Design review of the part built by this model. Coordinates are the model's own, in mm. Coordinates: 2 decimals unless noted, no trailing zeros. Loops run counter-clockwise (first coordinate to the right, second up) from the corner with the lowest first, then second, coordinate; pieces in that order, holes last. Notation, with made-up numbers: (8, 63.25) -> (38, 63.25) arc R21 ccw to (38, 88.25) -> close; hole circle Ø6 at (36.25, 60.5). An arc over 180 degrees is marked (long way). Answer as a JSON object with one key per item and string values.
Autodesk Inventor part; units mm, degrees
ref_plane "Начальная плоскость" through (0, 0, 0) normal (0, 0, 1) x (1, 0, 0)
ref_plane "Конечная плоскость" through (0, 0, 100) normal (0, 0, 1) x (1, 0, 0)
ref_plane "YZ Plane" through (0, 0, 0) normal (1, 0, 0) x (0, 1, 0)
ref_plane "Начальная плоскость" through (0, 0, 0) normal (0, 0, 1) x (1, 0, 0)
ref_plane "Конечная плоскость" through (0, 0, 100) normal (0, 0, 1) x (1, 0, 0)
sketch "Эскиз1" plane through (0, 0, 0) normal (0, 0, 1) x (1, 0, 0)
  line L0 (-14.4349, 0) -> (14.4349, 0)
  line L1 (0, -14) -> (0, 14)
  line L2 (0, 0) -> (7.5, 7.5) construction
  circle A0 centre (7.5, 7.5) radius 1.65 construction
  line L3 (5.85, 9.15) -> (9.15, 9.15)
  line L4 (9.15, 9.15) -> (9.15, 5.85)
  line L5 (9.15, 5.85) -> (5.85, 5.85)
  line L6 (5.85, 5.85) -> (5.85, 9.15)
  line L7 (3.235, 8.1636) -> (4.72, 9.9636)
  line L8 (4.7971, 10) -> (8.5, 10)
  line L9 (3.3121, 8) -> (4.95, 8)
  line L10 (4.95, 8) -> (4.95, 5.7985)
  line L11 (4.95, 5.7985) -> (2.6515, 3.5)
  line L12 (0, 3.5) -> (2.6515, 3.5)
  circle A1 centre (0, 0) radius 2.25
  line L13 (8.1636, 3.235) -> (9.9636, 4.72)
  line L14 (10, 4.7971) -> (10, 8.5)
  line L15 (8, 3.3121) -> (8, 4.95)
  line L16 (8, 4.95) -> (5.7985, 4.95)
  line L17 (5.7985, 4.95) -> (3.5, 2.6515)
  line L18 (3.5, 0) -> (3.5, 2.6515)
  arc A2 (10, 8.5) -> (8.5, 10) centre (8.5, 8.5) ccw
  line L19 (0, 0) -> (-7.5, 7.5) construction
  circle A3 centre (-7.5, 7.5) radius 1.65 construction
  line L20 (-5.85, 9.15) -> (-9.15, 9.15)
  line L21 (-9.15, 9.15) -> (-9.15, 5.85)
  line L22 (-9.15, 5.85) -> (-5.85, 5.85)
  line L23 (-5.85, 5.85) -> (-5.85, 9.15)
  line L24 (-3.235, 8.1636) -> (-4.72, 9.9636)
  line L25 (-4.7971, 10) -> (-8.5, 10)
  line L26 (-3.3121, 8) -> (-4.95, 8)
  line L27 (-4.95, 8) -> (-4.95, 5.7985)
  line L28 (-4.95, 5.7985) -> (-2.6515, 3.5)
  line L29 (0, 3.5) -> (-2.6515, 3.5)
  line L30 (-3.5, 0) -> (-3.5, 2.6515)
  line L31 (-5.7985, 4.95) -> (-3.5, 2.6515)
  line L32 (-8, 4.95) -> (-5.7985, 4.95)
  line L33 (-8, 3.3121) -> (-8, 4.95)
  line L34 (-8.1636, 3.235) -> (-9.9636, 4.72)
  line L35 (-10, 4.7971) -> (-10, 8.5)
  arc A4 (-8.5, 10) -> (-10, 8.5) centre (-8.5, 8.5) ccw
  line L36 (0, 14) -> (0, -14)
  line L37 (0, 0) -> (7.5, -7.5) construction
  circle A5 centre (7.5, -7.5) radius 1.65 construction
  line L38 (5.85, -9.15) -> (9.15, -9.15)
  line L39 (9.15, -9.15) -> (9.15, -5.85)
  line L40 (9.15, -5.85) -> (5.85, -5.85)
  line L41 (5.85, -5.85) -> (5.85, -9.15)
  line L42 (3.235, -8.1636) -> (4.72, -9.9636)
  line L43 (4.7971, -10) -> (8.5, -10)
  line L44 (3.3121, -8) -> (4.95, -8)
  line L45 (4.95, -8) -> (4.95, -5.7985)
  line L46 (4.95, -5.7985) -> (2.6515, -3.5)
  line L47 (0, -3.5) -> (2.6515, -3.5)
  line L48 (3.5, 0) -> (3.5, -2.6515)
  line L49 (5.7985, -4.95) -> (3.5, -2.6515)
  line L50 (8, -4.95) -> (5.7985, -4.95)
  line L51 (8, -3.3121) -> (8, -4.95)
  line L52 (8.1636, -3.235) -> (9.9636, -4.72)
  line L53 (10, -4.7971) -> (10, -8.5)
  arc A6 (8.5, -10) -> (10, -8.5) centre (8.5, -8.5) ccw
  line L54 (0, 0) -> (-7.5, -7.5) construction
  line L55 (-4.95, -8) -> (-4.95, -5.7985)
  line L56 (-3.3121, -8) -> (-4.95, -8)
  line L57 (-5.7985, -4.95) -> (-3.5, -2.6515)
  line L58 (-4.95, -5.7985) -> (-2.6515, -3.5)
  line L59 (-3.5, 0) -> (-3.5, -2.6515)
  line L60 (0, -3.5) -> (-2.6515, -3.5)
  circle A7 centre (-7.5, -7.5) radius 1.65 construction
  line L61 (-5.85, -5.85) -> (-5.85, -9.15)
  line L62 (-5.85, -9.15) -> (-9.15, -9.15)
  line L63 (-9.15, -9.15) -> (-9.15, -5.85)
  line L64 (-9.15, -5.85) -> (-5.85, -5.85)
  line L65 (-3.235, -8.1636) -> (-4.72, -9.9636)
  line L66 (-8, -4.95) -> (-5.7985, -4.95)
  line L67 (-8, -3.3121) -> (-8, -4.95)
  line L68 (-8.1636, -3.235) -> (-9.9636, -4.72)
  line L69 (-4.7971, -10) -> (-8.5, -10)
  line L70 (-10, -4.7971) -> (-10, -8.5)
  arc A8 (-10, -8.5) -> (-8.5, -10) centre (-8.5, -8.5) ccw
  arc A9 (3.235, 8.1636) -> (3.3121, 8) centre (3.3121, 8.1) ccw
  arc A10 (4.7971, 10) -> (4.72, 9.9636) centre (4.7971, 9.9) ccw
  arc A11 (8, 3.3121) -> (8.1636, 3.235) centre (8.1, 3.3121) ccw
  arc A12 (9.9636, 4.72) -> (10, 4.7971) centre (9.9, 4.7971) ccw
  arc A13 (-3.3121, 8) -> (-3.235, 8.1636) centre (-3.3121, 8.1) ccw
  arc A14 (-4.72, 9.9636) -> (-4.7971, 10) centre (-4.7971, 9.9) ccw
  arc A15 (-8.1636, 3.235) -> (-8, 3.3121) centre (-8.1, 3.3121) ccw
  arc A16 (-10, 4.7971) -> (-9.9636, 4.72) centre (-9.9, 4.7971) ccw
  arc A17 (-8, -3.3121) -> (-8.1636, -3.235) centre (-8.1, -3.3121) ccw
  arc A18 (-9.9636, -4.72) -> (-10, -4.7971) centre (-9.9, -4.7971) ccw
  arc A19 (-3.235, -8.1636) -> (-3.3121, -8) centre (-3.3121, -8.1) ccw
  arc A20 (-4.7971, -10) -> (-4.72, -9.9636) centre (-4.7971, -9.9) ccw
  arc A21 (4.72, -9.9636) -> (4.7971, -10) centre (4.7971, -9.9) ccw
  arc A22 (3.3121, -8) -> (3.235, -8.1636) centre (3.3121, -8.1) ccw
  arc A23 (8.1636, -3.235) -> (8, -3.3121) centre (8.1, -3.3121) ccw
  arc A24 (10, -4.7971) -> (9.9636, -4.72) centre (9.9, -4.7971) ccw
  point P0 (3.1, 8)
  point P1 (4.75, 10)
  point P2 (7.5, 9.15)
  point P3 (8, 3.1)
  point P4 (10, 4.75)
  point P5 (7.5, 5.85)
  point P6 (9.15, 7.5)
  point P7 (-3.1, 8)
  point P8 (-4.75, 10)
  point P9 (-7.5, 9.15)
  point P10 (-8, 3.1)
  point P11 (-10, 4.75)
  point P12 (-7.5, 5.85)
  point P13 (-9.15, 7.5)
  point P14 (3.1, -8)
  point P15 (4.75, -10)
  point P16 (7.5, -9.15)
  point P17 (8, -3.1)
  point P18 (10, -4.75)
  point P19 (7.5, -5.85)
  point P20 (9.15, -7.5)
  point P21 (-3.1, -8)
  point P22 (-7.5, -5.85)
  point P23 (-7.5, -9.15)
  point P24 (-9.15, -7.5)
  point P25 (-4.75, -10)
  point P26 (-8, -3.1)
  point P27 (-10, -4.75)
  dimension "d0" = 45
  dimension "d1" = 3.3
  dimension "d2" = 1.5
  dimension "d3" = 1.2
  dimension "d4" = 4.5
  dimension "d5" = 6.5
  dimension "d6" = 15
  dimension "d7" = 20
  dimension "d8" = 9.9
  dimension "d9" = 9.5
  dimension "d10" = 6.2
  dimension "d11" = 2
  dimension "d18" = 0.1
  dimension "d19" = 0.1
extrude "Тело" add sketch "Эскиз1" along normal up to surface (100 mm away) from surface at 0 contours A1 L1 L12 L11 L10 L9 A9 L7 A10 L8 A2 L14 A12 L13 A11 L15 L16 L17 L18 L0 | L0 L48 L49 L50 L51 A23 L52 A24 L53 A6 L43 A21 L42 A22 L44 L45 L46 L47 L1 A1 | A1 L0 L30 L31 L32 L33 A15 L34 A16 L35 A4 L25 A14 L24 A13 L26 L27 L28 L29 L1 | L1 L60 L58 L55 L56 A19 L65 A20 L69 A8 L70 A18 L68 A17 L67 L66 L57 L59 L0 A1
sketch "Эскиз2" plane through (0, 0, 0) normal (0, 0, 1) x (1, 0, 0)
  line L0 (0, 0) -> (10, 0)
ref_plane "РабПлоскость3" through (0, 0, 0) normal (0, -1, 0) x (1, 0, 0)
sketch "Эскиз3" plane through (0, 0, 0) normal (0, -1, 0) x (1, 0, 0)
  line L0 (-2, 0) -> (12, 0)
  line L1 (-2, 100) -> (12, 100)
  dimension "d25" = 100
equation "\"G_OFFSET_START\" = 0"
equation "\"G_OFFSET_END\" = 0"
properties part number "короткая палка"
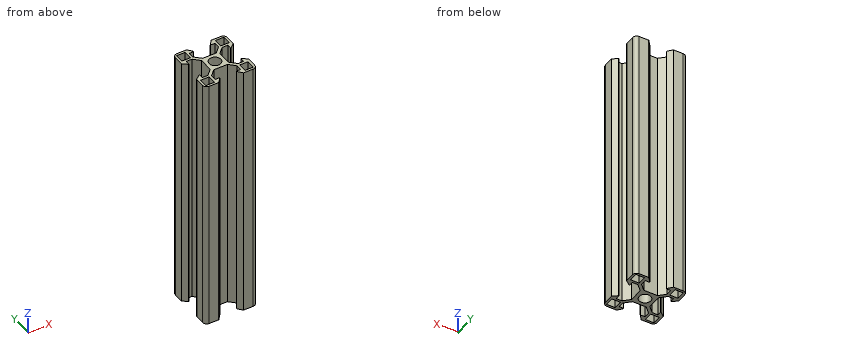
1) Add section A-A, the plane y = 7. Give the boundary of the cut face in (x, z), and give its area (3 significant figures).
Completed:
{"outline": "(-10, 0) -> (-9.15, 0) -> (-9.15, 100) -> (-10, 100) -> close; (-5.85, 0) -> (-4.95, 0) -> (-4.95, 100) -> (-5.85, 100) -> close; (4.95, 0) -> (5.85, 0) -> (5.85, 100) -> (4.95, 100) -> close; (9.15, 0) -> (10, 0) -> (10, 100) -> (9.15, 100) -> close", "area": "350 mm²"}
2) Add section B-B, the plane x = 0. Give the boundary of the cut face in (y, z).
Completed:
{"outline": "(-3.5, 0) -> (-2.25, 0) -> (-2.25, 100) -> (-3.5, 100) -> close; (2.25, 0) -> (3.5, 0) -> (3.5, 100) -> (2.25, 100) -> close"}
3) Wall thickness on probe 1 along X at (y, z) = (-7, 56); probe 2 along X at (y, z) = (0, 44): over which ranges is each line inside the solid? List them lowest first.
Completed:
{"probe 1": "-10 to -9.15, -5.85 to -4.95, 4.95 to 5.85, 9.15 to 10", "probe 2": "-3.5 to -2.25, 2.25 to 3.5"}
4) Clearance check with flat-ended pins moving along their axes: pin 1 Ø4 at (y, z) = (0, 27.5) entering from +X; pin 2 Ø1.8 at (x, z) = (-3.5, 30.5) entering from -Y; pin 3 Ø2 at (x, z) = (-1.5, 77) entering from +Y. State where each tip first meets the part, or that it passes through.
Completed:
{"pin 1": "x = 3.5", "pin 2": "y = -9.58", "pin 3": "y = 3.5"}
5) Add section D-D, the plane z = 18.5. Count the separate pieces of the cut face and the enclosed holes in it, and give its area (3 significant figures).
Completed:
{"separate pieces": "1", "enclosed holes": "5", "area": "119 mm²"}
